from build123d import *

# Parameters (mm, degrees)
SKETCH1_R           = 5.08
BOSS_EXTRUDE1_DEPTH = 2.116666667
SKETCH2_R           = 6.6675
SKETCH2_R_2         = 5.08
BOSS_EXTRUDE2_DEPTH = 1.5875


with BuildPart() as part:
    # Sketch1 → Boss-Extrude1 (new body)
    with BuildSketch(Plane(origin=(0, 0, 0), x_dir=(1, 0, 0), z_dir=(0, 1, 0))):
        with BuildLine():
            Line((-25.4, 50.8), (-20.32, 50.8))
            Line((-20.32, 50.8), (11.43, 43.486136085))
            ThreePointArc((11.43, 43.486136085), (23.688747156, 36.694883241), (30.48, 24.436136085))
            Line((30.48, 24.436136085), (38.06337105, -13.663863915))
            ThreePointArc((38.06337105, -13.663863915), (34.032755304, -22.014801976), (25.4, -25.4))
            Line((25.4, -25.4), (-25.4, -25.4))
            ThreePointArc((-25.4, -25.4), (-34.380256121, -21.680256121), (-38.1, -12.7))
            Line((-38.1, -12.7), (-38.1, 38.1))
            ThreePointArc((-38.1, 38.1), (-34.380256121, 47.080256121), (-25.4, 50.8))
        make_face()
        with Locations((11.43, 24.436136085)):
            Circle(SKETCH1_R, mode=Mode.SUBTRACT)
    extrude(amount=BOSS_EXTRUDE1_DEPTH)

    # Sketch2 → Boss-Extrude2 (add)
    with BuildSketch(Plane(origin=(0, 2.116666667, 0), x_dir=(1, 0, 0), z_dir=(0, 1, 0))):
        with Locations((11.43, 24.436136085)):
            Circle(SKETCH2_R)
        with Locations((11.43, 24.436136085)):
            Circle(SKETCH2_R_2, mode=Mode.SUBTRACT)
    extrude(amount=BOSS_EXTRUDE2_DEPTH)


solid = part.part
Work out the finished part from the listing and answer in its coordinate system (mm). A direction names the side the tool comes from. Coordinates: 2 decimals unless noted, no trailing zeros. Write each loop counter-clockwise with the first axis right and the second up, starting at its lowest first coordinate (ties: lowest second). Pieces come first, ordered by that corner, then holes. Notation, with made-up numbers: M 28.25,86.5 L 83.25,86.5 A22 ccw 83.25,97.5 Z; hole C 37,48.5 d8. An arc over 180 degrees is marked long. Write item = value, one per line.
1. The part is cut by section B-B (y = 2.9). Determine the outline of the cut face in (x, z) (1 decimal).
Solution:
outline = C 11.4,-24.4 d13.3; hole C 11.4,-24.4 d10.2
2. Determine the mould class of faces 1 (the face through (23.55, 1.04, -36.83)), 2 (the face through (-38.1, 1, -12)), 3 (the face through (10.769, 1.826, -29.473)) for opening direction X: released by +X, released by -X, zero draft, split by the parting line, or undercut.
Solution:
face_1 = released by +X
face_2 = released by -X
face_3 = undercut
3. For faces 4 (the face through (-23, 1, -50.8)), 5 (the face through (14.507, 2.899, -18.521)), determine the directions among +Z, -Z, +X, -X, +Y, -Y from which every point of the face is accessible in a straight line to the end or side of a thin tool.
Solution:
face_4 = -Z, +X, -X, +Y, -Y
face_5 = +Y
4. Straight lines are drawn through the part: line 1 (Z direction, x = 11.43, y = 2.3); line 2 (Z direction, x = 11.43, y = 0.9); line 3 (Y direction, x = 22, z = 5.5). For each, find the intervals that lie inside material, in ascending order. Write a range as from..to.
Solution:
line_1 = -31.1..-29.52, -19.36..-17.77
line_2 = -43.49..-29.52, -19.36..25.4
line_3 = 0..2.12
5. The part is cut by section A-A (x = 15). Determine the outline of the cut face in (y, z), then the cut area to 3 significant figures.
Solution:
outline = M 0,-42.38 L 2.12,-42.38 L 2.12,-30.07 L 3.7,-30.07 L 3.7,-28.05 L 0,-28.05 Z; M 0,-20.82 L 3.7,-20.82 L 3.7,-18.8 L 2.12,-18.8 L 2.12,25.4 L 0,25.4 Z
area = 135 mm2
6. Flat-ended cylindrical pins translate along their axes: pin 1 (23 mm diameter, centred on x = -11, z = -15.5, fed in from +Y); pin 2 (2 mm diameter, centred on x = -29, y = 2, fed in from -Z). Find the tip coordinate at first contact, or state that the pin passes through.
Solution:
pin_1 = 2.12
pin_2 = -50.53
7. The part is cut by section D-D (x = 32.5). Determine the outline of the cut face in (y, z).
Solution:
outline = M 0,-14.29 L 2.12,-14.29 L 2.12,23.23 L 0,23.23 Z
8. The part is cut by section C-C (z = -35.5). Determine the outline of the cut face in (x, y).
Solution:
outline = M -38.1,0 L 24.81,0 L 24.81,2.12 L -38.1,2.12 Z
